```python
from build123d import *
from build123d import SkipClean  # not in build123d's __all__

# Parameters (mm, degrees)
F2_SIZE   = 0.5
F4_DEPTH  = 8
F6_DEPTH  = 4
F7_R      = 4
F8_DEPTH  = 9.5
F10_D     = 3.2
F10_DEPTH = 14
F10_TIP   = 0.9613769904
F11_R     = 1.6
F12_DEPTH = 2.53


# Not quite as in the source:
# - after a boolean that leaves OpenCascade's solid faulty, fix() repairs it


with BuildPart() as f1:
    # F0 (on Front) → F1 (revolve)
    with BuildSketch(Plane.XZ):
        Polygon((-2, 0), (0, 0), (0, 24.5), (-4, 24.5), (-4, 12), (-2, 12), align=None)
    revolve(axis=Axis((0, 0, 12.25), (0, 0, -1)))

    # F2
    f2_edges = [f1.edges().sort_by_distance(p)[0] for p in [
        (2, 0, 0),
    ]]
    chamfer(f2_edges, length=F2_SIZE)

    # F3 (on face) → F4 (join)
    with BuildSketch(Plane.XY.offset(24.5)):
        with BuildLine():
            Line((-3.1224989992, -2.5), (3.1224989992, -2.5))
            ThreePointArc((3.1224989992, -2.5), (3.7742546282, -1.3247648854), (4, 0))
            ThreePointArc((4, 0), (-1.3247648854, 3.7742546282), (-3.1224989992, -2.5))
        make_face()
    with SkipClean():  # cleaning this boolean's faces spoils the solid; the shape is the same uncleaned
        extrude(amount=F4_DEPTH)

    # F5 (on face) → F6 (join)
    with BuildSketch(Plane.XY.offset(32.5)):
        with BuildLine():
            Line((-3.1224989992, -2.5), (3.1224989992, -2.5))
            ThreePointArc((3.1224989992, -2.5), (3.8760324942, -0.9881154306), (3.9382737335, 0.7))
            Line((3.9382737335, 0.7), (2.1, 2.5))
            Line((2.1, 2.5), (-2.1, 2.5))
            Line((-2.1, 2.5), (-3.7080992435, 1.5))
            ThreePointArc((-3.7080992435, 1.5), (-3.9578110223, -0.5794237754), (-3.1224989992, -2.5))
        make_face()
    extrude(amount=F6_DEPTH)

    add(f1.part.fix(), mode=Mode.REPLACE)

    # F7 (on face) → F8 (join)
    with BuildSketch(Plane.XY.offset(36.5)):
        Circle(F7_R)
    extrude(amount=F8_DEPTH)

    # F10
    with Locations(Plane.XY.offset(46)):
        with Locations((0, 0)):
            Hole(F10_D / 2, depth=F10_DEPTH)
            with Locations((0, 0, -(F10_DEPTH + F10_TIP / 2))):  # 118° drill point
                Cone(0, F10_D / 2, F10_TIP, mode=Mode.SUBTRACT)

    # F11 (on face) → F12 (cut)
    with BuildSketch(Plane(origin=(0, 2.5, 0), x_dir=(-1, 0, 0), z_dir=(0, 1, 0))):
        with Locations((0, 34.5)):
            Circle(F11_R)
    extrude(amount=-F12_DEPTH, mode=Mode.SUBTRACT)


solid = f1.part
```
Part model, mm, in its own coordinate system. A direction names the side the tool comes from. Round coordinates to 2 decimals unless told otherwise and drop trailing zeros. Write each loop counter-clockwise with the first axis right and the second up, starting at its lowest first coordinate (ties: lowest second). Pieces come first, ordered by that corner, then holes.
Item 1: Probe L1, parallel to Y at x = 0, z = 40.5; L2, parallel to Z at x = 0.75, y = 3.25; L3, parallel to Z at x = -1, y = -3.25. List the from-to ranges inside material, lowest first.
Results:
L1: y = -4 to -1.6, 1.6 to 4
L2: z = 12 to 32.5, 36.5 to 46
L3: z = 12 to 24.5, 36.5 to 46
Item 2: Two-plate mould, pull along Z, no slides. Class faces 5 (the flat face through (2, 0, 46)), 6 (the flat face through (0, 3, 36.5)), 7 (the flat face through (0, 0, 0)): +Z half, -Z half, draft (parallel to the pull), parting line (faces both ways), or undercut.
Results:
face 5: +Z half
face 6: undercut
face 7: -Z half
Item 3: Which spindle directions (+Z, -Z, +X, -X, +Y, -Y) get a long thin tool onto all of the face, cutting with end or side? Do faces 1 (the flat face through (-2.89, 2.01, 34.47)), 2 (the cylindrical face through (0.35, -1.56, 38.9)), 3 (the flat face through (2, -1, 12)), 4 (the cylindrical face through (1.27, 1.55, 33.53)). Say none if no direction does.
Results:
face 1: -X, +Y
face 2: +Z
face 3: -Z
face 4: +Y
Item 4: Cut at A-A, the plane y = 3.5. Give the cut face in (x, z).
Results:
outline: (-1.94, 12) - (1.94, 12) - (1.94, 32.5) - (-1.94, 32.5) - close; (-1.94, 36.5) - (1.94, 36.5) - (1.94, 46) - (-1.94, 46) - close
Item 5: Drop flat-ended pins along their axis: pin 1 Ø1.5 at (x, z) = (3, 10) entering from +Y; pin 2 Ø1 at (x, z) = (-0.5, 5) entering from -Y; pin 3 Ø3 at (x, z) = (1, 32) entering from -Y; pin 4 Ø1 at (x, y) = (0.5, 0.5) entering from +Z. Give the stop position or say it passes through.
Results:
pin 1: passes through
pin 2: stops at y = -2
pin 3: stops at y = -2.5
pin 4: stops at z = 31.76
Item 6: Cut at B-B, the plane z = 22.5. Give the cut face in (x, y), plus the area to 3 significant figures.
Results:
outline: circle Ø8 at (0, 0)
area: 50.3 mm2
Item 7: Cut at C-C, the plane x = 2.5. Give the cut face in (y, z).
Results:
outline: (-3.12, 12) - (3.12, 12) - (3.12, 32.5) - (2.11, 32.5) - (2.11, 36.5) - (3.12, 36.5) - (3.12, 46) - (-3.12, 46) - (-3.12, 36.5) - (-2.5, 36.5) - (-2.5, 24.5) - (-3.12, 24.5) - close
Item 8: Cut at D-D, the plane z = 11.5. Give the cut face in (x, y), plus the area to 3 significant figures.
Results:
outline: circle Ø4 at (0, 0)
area: 12.6 mm2
